from build123d import *

# Parameters (mm, degrees)
SKETCH1_R           = 2.55
BOSS_EXTRUDE1_DEPTH = 2
SKETCH2_R           = 1.25
BOSS_EXTRUDE2_DEPTH = 25
SKETCH3_W           = 6
SKETCH3_H           = 1
CUT_EXTRUDE1_DEPTH  = 1


with BuildPart() as part:
    # Sketch1 → Boss-Extrude1 (new body)
    with BuildSketch(Plane(origin=(0, 0, 0), x_dir=(1, 0, 0), z_dir=(0, 1, 0))):
        Circle(SKETCH1_R)
    extrude(amount=BOSS_EXTRUDE1_DEPTH)

    # Sketch2 → Boss-Extrude2 (add)
    with BuildSketch(Plane(origin=(0, 0, 0), x_dir=(1, 0, 0), z_dir=(0, 1, 0))):
        Circle(SKETCH2_R)
    extrude(amount=-BOSS_EXTRUDE2_DEPTH)

    # Sketch3 → Cut-Extrude1 (cut)
    with BuildSketch(Plane(origin=(0, 2, 0), x_dir=(1, 0, 0), z_dir=(0, 1, 0))):
        Rectangle(SKETCH3_W, SKETCH3_H)
    extrude(amount=-CUT_EXTRUDE1_DEPTH, mode=Mode.SUBTRACT)


solid = part.part
Could you check a few things on this model? Use its own coordinates, in mm. A direction names the side the tool comes from. Coordinates: 2 decimals unless noted, no trailing zeros. Order: outer loops, then holes, each group sorted by start corner. A loop starts at its lowest first (then second) coordinate and runs counter-clockwise, first axis right, second up. Notation, with made-up numbers: (17, -16) - (44, -16) arc R17 cw to (44, 11) - close; hole circle Ø10 at (-4.75, -1). An arc over 180 degrees is marked (long way). Answer in a Markdown table with one row per item. Add a question column.
(1) If we section it at C-C, the plane y = -14.25: Please give me the cut outline in (x, z), then the cut area to 3 significant figures.
(2) On a 3-axis mill with a long thin cutter (end or side, diameter ignored), from which of +Z, -Z, +X, -X, +Y, -Y can I reach the whole of each face in a straight line? I mean faces 1 (the face through (0, 2, -1)), 2 (the face through (1, 0, -1)), 3 (the face through (0, 1.5, -0.5)). Say none if no direction works.
(3) If we section it at A-A, the plane z = 0: Please give me the cut outline in (x, y), then the cut area to 3 significant figures.
(4) I need wall thicknesses on L1, parallel to Y at x = 2.05, z = -1.2; L2, parallel to X at y = -0.5, z = -0.1; L3, parallel to Y at x = -2.3, z = -0.3. Which ranges of each line are inside material? Lowest first, please.
(5) If we section it at D-D, the plane x = -0.55: Please give me the cut outline in (y, z).
(6) If we section it at B-B, the plane x = 1.85: Please give me the cut outline in (y, z) (3 decimals).
(7) If we mould it in two halves opening along Z, with no side actions, what happens to faces 4 (the face through (0, -25, 0)), 5 (the face through (-0.27, -12.32, 1.22)), 6 (the face through (0, 1, 0))? For each: released by +Z, released by -Z, zero draft, split by the parting line, or undercut.
(8) Will these pins go through, and if not, where does the flat tip stop? pin 1 (0.5 mm diameter, centred on x = 0, z = 0, fed in from +Y); pin 2 (3 mm diameter, centred on x = -0.5, y = -10, fed in from -Z); pin 3 (2 mm diameter, centred on y = -8, z = -1.5, fed in from -X).
Results are:
| question | item | result |
|---|---|---|
| 1 | outline | circle Ø2.5 at (0, 0) |
| 1 | area | 4.91 mm2 |
| 2 | face 1 | +Z, -Z, +X, -X, +Y |
| 2 | face 2 | -Y |
| 2 | face 3 | +X, -X, +Y |
| 3 | outline | (-2.55, 0) - (-1.25, 0) - (-1.25, -25) - (1.25, -25) - (1.25, 0) - (2.55, 0) - (2.55, 1) - (-2.55, 1) - close |
| 3 | area | 67.6 mm2 |
| 4 | L1 | y = 0 to 2 |
| 4 | L2 | x = -1.25 to 1.25 |
| 4 | L3 | y = 0 to 1 |
| 5 | outline | (-25, -1.12) - (0, -1.12) - (0, -2.49) - (2, -2.49) - (2, -0.5) - (1, -0.5) - (1, 0.5) - (2, 0.5) - (2, 2.49) - (0, 2.49) - (0, 1.12) - (-25, 1.12) - close |
| 6 | outline | (0, -1.755) - (2, -1.755) - (2, -0.5) - (1, -0.5) - (1, 0.5) - (2, 0.5) - (2, 1.755) - (0, 1.755) - close |
| 7 | face 4 | zero draft |
| 7 | face 5 | split by the parting line |
| 7 | face 6 | undercut |
| 8 | pin 1 | stops at y = 1 |
| 8 | pin 2 | stops at z = -1.25 |
| 8 | pin 3 | stops at x = -1.15 |
